```python
from build123d import *

# Parameters (mm, degrees)
EXTRUDE1_DEPTH = 8
EXTRUDE2_DEPTH = 8
SKETCH3_R      = 1.95
EXTRUDE3_DEPTH = 15
SKETCH4_R      = 1.95
EXTRUDE4_DEPTH = 10
SKETCH5_R      = 1.95
EXTRUDE5_DEPTH = 10


with BuildPart() as part:
    # Sketch1 → Extrude1 (new body)
    with BuildSketch(Plane.XY):
        Polygon((-45.778459293, 10.844789824), (-35.257703973, 10.844789824), (-35.257703973, 15.844789824), (14.742296027, 15.844789824), (14.742296027, 10.844789824), (25.221540707, 10.844789824), (25.221540707, -19.155210176), (-45.778459293, -19.155210176), align=None)
    extrude(amount=EXTRUDE1_DEPTH)

    # Sketch2 → Extrude2 (cut)
    with BuildSketch(Plane.XY.offset(8)):
        with BuildLine():
            Line((-45.778459293, -19.155210176), (25.221540707, -19.155210176))
            add(Edge.make_bspline(
                [(-45.778459293, -19.155210176), (-33.94270631, -13.318817895), (-10.275364533, -1.648086759), (13.390626945, -13.320186926), (25.221540707, -19.155210176)],
                knots=[0, 0, 0, 0, 0.500087973, 1, 1, 1, 1], degree=3))
        make_face()
    extrude(amount=-EXTRUDE2_DEPTH, mode=Mode.SUBTRACT)

    # Sketch3 → Extrude3 (cut)
    with BuildSketch(Plane(origin=(0, 15.844789824, 0), x_dir=(-1, 0, 0), z_dir=(0, 1, 0))):
        with Locations((22.757703973, 4)):
            Circle(SKETCH3_R)
        with Locations((-2.242296027, 4)):
            Circle(SKETCH3_R)
    extrude(amount=-EXTRUDE3_DEPTH, mode=Mode.SUBTRACT)

    # Sketch4 → Extrude4 (cut)
    with BuildSketch(Plane(origin=(25.221540707, 0, 0), x_dir=(0, 0, -1), z_dir=(1, 0, 0))):
        with Locations((-4, 2.844789824)):
            Circle(SKETCH4_R)
        with Locations((-4, -12.155210176)):
            Circle(SKETCH4_R)
    extrude(amount=-EXTRUDE4_DEPTH, mode=Mode.SUBTRACT)

    # Sketch5 → Extrude5 (cut)
    with BuildSketch(Plane.ZY.offset(45.778459293)):
        with Locations((4, 2.844789824)):
            Circle(SKETCH5_R)
        with Locations((4, -12.155210176)):
            Circle(SKETCH5_R)
    extrude(amount=-EXTRUDE5_DEPTH, mode=Mode.SUBTRACT)


solid = part.part
```
Source: CAD feature listing. Evaluate the final solid. Frame: model axes, mm. A direction names the side the tool comes from. Coordinates: 2 decimals unless noted, no trailing zeros. Write each loop counter-clockwise with the first axis right and the second up, starting at its lowest first coordinate (ties: lowest second). Pieces come first, ordered by that corner, then holes. Notation, with made-up numbers: (60, 77) - (103, 77) arc R17 cw to (103, 106) - close; hole circle Ø8 at (-7.75, -39). An arc over 180 degrees is marked (long way). Answer as a JSON object with one key per item and string values.
Q1. Draft query along Y for faces 6 (the flat face through (20, 10.845, 4)), 7 (the flat face through (-10, 2, 8)), 8 (the cylindrical face through (-40.8, -10.8, 2.6)). Return one class per face: released by +Y, released by -Y, zero draft, split by the parting line, or undercut.
Ans:
{"face 6": "released by +Y", "face 7": "zero draft", "face 8": "undercut"}
Q2. Set-up query: faces 1 (the flat face through (-35.258, 13, 4)), 2 (the flat face through (15.222, -12, 4)), 3 (the flat face through (14.742, 13, 4)), 4 (the flat face through (-35.778, -12, 4)), 5 (the flat face through (-23, 0.845, 4)). Return all of +Z, -Z, +X, -X, +Y, -Y with unobstructed straight access to the full face (end or side cutting, diameter ignored); none if empty.
Ans:
{"face 1": "+Z, -Z, -X, +Y", "face 2": "+X", "face 3": "+Z, -Z, +X, +Y", "face 4": "-X", "face 5": "+Y"}
Q3. Material intervals for line 1 (X direction, y = 12.5, z = 4.25); line 2 (Y direction, x = -43.25, z = 4); line 3 (X direction, y = 12.5, z = 5.5), sorted ascending. Write a range as [from, to].
Ans:
{"line 1": "x = [-35.26, -24.69], [-20.82, 0.31], [4.18, 14.74]", "line 2": "y = [-17.91, -14.11], [-10.21, 0.89], [4.79, 10.84]", "line 3": "x = [-35.26, -24], [-21.51, 1], [3.49, 14.74]"}
Q4. Section query B-B, the plane y = 6.5. Output: boundary loops of the cut face in (x, z), plus the area to 3 significant figures.
Ans:
{"outline": "(-45.78, 0) - (25.22, 0) - (25.22, 8) - (-45.78, 8) - close; hole circle Ø3.9 at (-22.76, 4); hole circle Ø3.9 at (2.24, 4)", "area": "544 mm2"}
Q5. First-contact query: pin 1 Ø1.2 at (x, z) = (2.5, 4.5) entering from +Y; pin 2 Ø1.2 at (y, z) = (2.5, 4) entering from -X; pin 3 Ø2 at (x, y) = (-20, -4) entering from -Z; pin 4 Ø1.5 at (y, z) = (14, 5.5) entering from -X. Flat tips, straight axial feed; report the tip coordinate or a pass-through.
Ans:
{"pin 1": "stops at y = 0.84", "pin 2": "stops at x = -35.78", "pin 3": "stops at z = 0", "pin 4": "stops at x = -35.26"}
Q6. Section query A-A, the plane y = 12.5. Output: boundary loops of the cut face in (x, z), plus the area to 3 significant figures.
Ans:
{"outline": "(-35.26, 0) - (14.74, 0) - (14.74, 8) - (-35.26, 8) - close; hole circle Ø3.9 at (-22.76, 4); hole circle Ø3.9 at (2.24, 4)", "area": "376 mm2"}
